from build123d import *


with BuildPart() as f1:
    # F0 (on Front) → F1 (revolve)
    with BuildSketch(Plane.XZ):
        with BuildLine():
            Line((0, 28.575), (0, 0))
            Line((0, 0), (3.81, 0))
            Line((3.81, 0), (3.81, 17.78))
            ThreePointArc((3.81, 17.78), (4.739936, 20.025064), (6.985, 20.955))
            Line((6.985, 20.955), (21.43125, 20.955))
            ThreePointArc((21.43125, 20.955), (21.992516, 21.187484), (22.225, 21.74875))
            Line((22.225, 21.74875), (22.225, 23.33625))
            ThreePointArc((22.225, 23.33625), (21.992516, 23.897516), (21.43125, 24.13))
            Line((21.43125, 24.13), (3.175, 24.13))
            Line((3.175, 24.13), (3.175, 28.575))
            Line((3.175, 28.575), (0.79375, 28.575))
            Line((0.79375, 28.575), (0, 28.575))
        make_face()
    revolve(axis=Axis((1.905, 0, 0), (1, 0, 0)))


solid = f1.part
Build history of the part. All positions in model axes, mm. A direction names the side the tool comes from. Coordinates: 2 decimals unless noted, no trailing zeros. Write each loop counter-clockwise with the first axis right and the second up, starting at its lowest first coordinate (ties: lowest second). Pieces come first, ordered by that corner, then holes.
(1) Pin check, flat tips, straight feed: pin 1 Ø6 at (x, z) = (3, -8.5) entering from +Y; pin 2 Ø2 at (x, z) = (17.5, -16) entering from +Y; pin 3 Ø2 at (x, y) = (8.5, 4) entering from -Z. Stop position of each tip, or through.
(2) 3-axis set-ups, long thin cutter, end or side, ignore diameter. For faces 4 (the flat face through (3.175, 21, 13)), 5 (the cylindrical face through (1.565, -1.256, -28.547)): which of +Z, -Z, +X, -X, +Y, -Y reach the whole face in a straight line?
(3) Cut at C-C on x = 12.5. List the corners of the cut face in (y, z) (3 decimals).
(4) Drill centre lines: line 1 (Y direction, x = 11, z = 0) (3 decimals); line 2 (Z direction, x = 20, y = 17). Where is each one in solid material? Low to high.
(5) Cut at D-D on x = 1.75. List the corners of the cut face in (y, z) (3 decimals), and give its area (3 significant figures).
(6) Mould opens along Y. For faces 1 (the cylindrical face through (12.175, -7.248, 23.016)), 2 (the flat face through (3.81, 0, 0)), 3 (the flat face through (22.225, 21, 7)) say: pulls with the +Y half, pulls with the -Y half, needs draft (parallel to the pull), parting line crosses it, or undercut.
Working result:
1. pin 1: stops at y = 28.04
1. pin 2: stops at y = 18.9
1. pin 3: stops at z = -23.94
2. face 4: +X
2. face 5: +X, -X
3. outline: circle Ø48.26 at (0, 0); hole circle Ø41.91 at (0, 0)
4. line 1: y = -24.13 to -20.955, 20.955 to 24.13
4. line 2: z = -17.12 to -12.25, 12.25 to 17.12
5. outline: circle Ø57.15 at (0, 0)
5. area: 2,570 mm2
6. face 1: parting line crosses it
6. face 2: undercut
6. face 3: needs draft
